The listing builds one solid part. Answer for the finished solid, in the listing's coordinates (mm). A direction names the side the tool comes from. Give positions to 0.01 mm unless a question says otherwise; leave off trailing zeros. Loops run counter-clockwise (first coordinate to the right, second up) from the corner with the lowest first, then second, coordinate; pieces in that order, holes last. Notation, with made-up numbers: (27.25, -1.75) - (86.25, -1.75) arc R17 ccw to (86.25, 16.25) - close; hole circle Ø5 at (35, 81). An arc over 180 degrees is marked (long way). One line per item, written item: value. Start each with the question number.
from build123d import *

# Parameters (mm, degrees)
CYLINDER026_R     = 1.75
CYLINDER026_DEPTH = 20
CYLINDER025_R     = 1.75
CYLINDER025_DEPTH = 20
CYLINDER014_R     = 1.2
CYLINDER014_DEPTH = 10
CYLINDER013_R     = 1.2
CYLINDER013_DEPTH = 10
SKETCH_R          = 4
PAD_DEPTH         = 3
BOX008_W          = 23.5
BOX008_H          = 12.5
BOX008_DEPTH      = 10
BOX007_W          = 32.5
BOX007_H          = 12.5
BOX007_DEPTH      = 2
BOX006_W          = 40.5
BOX006_H          = 20.5
BOX006_DEPTH      = 9.5


with BuildPart() as cylinder061:
    # Cylinder026 → Cylinder026 (new body)
    with BuildSketch(Plane(origin=(40, -18, 77), x_dir=(1, 0, 0), z_dir=(0, 0, 1))):
        Circle(CYLINDER026_R)
    extrude(amount=CYLINDER026_DEPTH)


with BuildPart() as cylinder060:
    # Cylinder025 → Cylinder025 (new body)
    with BuildSketch(Plane(origin=(28, -18, 77), x_dir=(1, 0, 0), z_dir=(0, 0, 1))):
        Circle(CYLINDER025_R)
    extrude(amount=CYLINDER025_DEPTH)


with BuildPart() as cylinder049:
    # Cylinder014 → Cylinder014 (new body)
    with BuildSketch(Plane(origin=(55, 19, -5), x_dir=(1, 0, 0), z_dir=(0, 0, 1))):
        Circle(CYLINDER014_R)
    extrude(amount=CYLINDER014_DEPTH)


with BuildPart() as cylinder048:
    # Cylinder013 → Cylinder013 (new body)
    with BuildSketch(Plane(origin=(55, -9.5, -5), x_dir=(1, 0, 0), z_dir=(0, 0, 1))):
        Circle(CYLINDER013_R)
    extrude(amount=CYLINDER013_DEPTH)


with BuildPart() as tapa:
    # Sketch → Pad (new body)
    with BuildSketch(Plane.XY.offset(-3)):
        with BuildLine():
            ThreePointArc((13.733879, 10.914307), (6.136168, -2.245404), (17.776624, -12.012848))
            Line((17.776624, -12.012848), (97.776624, -12.012848))
            ThreePointArc((97.776624, -12.012848), (119.712869, 11.926287), (93.95296, 31.692625))
            Line((13.733879, 10.914307), (93.95296, 31.692625))
        make_face()
        with Locations((17.77659, -0.192848)):
            Circle(SKETCH_R, mode=Mode.SUBTRACT)
        with Locations((97.776659, 10.007152)):
            Circle(SKETCH_R, mode=Mode.SUBTRACT)
    extrude(amount=PAD_DEPTH)


with BuildPart() as cube008:
    # Box008 → Box008 (new body)
    with BuildSketch(Plane(origin=(8.5, 4, 0), x_dir=(1, 0, 0), z_dir=(0, 0, 1))):
        with Locations((11.75, 6.25)):
            Rectangle(BOX008_W, BOX008_H)
    extrude(amount=BOX008_DEPTH)


with BuildPart() as cube007:
    # Box007 → Box007 (new body)
    with BuildSketch(Plane(origin=(4, 4, 0), x_dir=(1, 0, 0), z_dir=(0, 0, 1))):
        with Locations((16.25, 6.25)):
            Rectangle(BOX007_W, BOX007_H)
    extrude(amount=BOX007_DEPTH)


with BuildPart() as tapa_izquierda_interior:
    # Box006 → Box006 (new body)
    with BuildSketch(Plane.XY):
        with Locations((20.25, 10.25)):
            Rectangle(BOX006_W, BOX006_H)
    extrude(amount=BOX006_DEPTH)

    # Cut008: cut Cube007
    add(cube007.part, mode=Mode.SUBTRACT)

    # Cut009: cut Cube008
    add(cube008.part, mode=Mode.SUBTRACT)


with BuildPart() as tapa_izquierda_interior_1:
    # Cut009 placement: moved
    add(tapa_izquierda_interior.part.moved(Location((72.5, 0, -12.5))))

    # Fusion006: union Tapa
    add(tapa.part)


with BuildPart() as tapa_izquierda_interior_2:
    # Fusion006 placement: moved
    add(tapa_izquierda_interior_1.part.moved(Location((0, 0, -0.5))))

    # Cut013: cut Cylinder048
    add(cylinder048.part, mode=Mode.SUBTRACT)

    # Cut014: cut Cylinder049
    add(cylinder049.part, mode=Mode.SUBTRACT)


with BuildPart() as tapa_izquierda_interior_3:
    # Cut014 placement: moved
    add(tapa_izquierda_interior_2.part.moved(Location((-21, -19, 89))))

    # Cut049: cut Cylinder060
    add(cylinder060.part, mode=Mode.SUBTRACT)

    # Cut050: cut Cylinder061
    add(cylinder061.part, mode=Mode.SUBTRACT)


solid = tapa_izquierda_interior_3.part
1. A cutting plane is placed at B-B (x = 34). Determine the outline of the cut face in (y, z).
2. Flat-ended cylindrical pins translate along their axes: pin 1 (5 mm diameter, centred on x = 71, z = 80.5, fed in from +Y); pin 2 (6 mm diameter, centred on y = -24.5, z = 86, fed in from -X); pin 3 (3 mm diameter, centred on y = -19, z = 83, fed in from -X). Find the tip coordinate at first contact, or state that the pin passes through.
3. Determine the mould class of faces 1 (the flat face through (32.282, 2.158, 86.979)), 2 (the cylindrical face through (40.9, -16.5, 87)), 3 (the cylindrical face through (72.78, -8.82, 86.98)), 4 (the flat face through (36, -31.013, 87)) for opening direction X: released by +X, released by -X, zero draft, split by the parting line, or undercut.
4. A cutting plane is placed at A-A (z = 80). Determine the outline of the cut face in (x, y), plus the area to 4 significant figures.
5. Find the intervals of material crossed by L1, parallel to X at y = -18, z = 86.35; L2, parallel to Y at x = 34, z = 86.6; L3, parallel to Y at x = 78, z = 77.25, in increasing order. Write a range as [from, to].
6. For faces 5 (the flat face through (51.5, -9, 81)), 6 (the cylindrical face through (-14.9, -21.02, 86.98)), 7 (the flat face through (71, 1.5, 81)), 8 (the flat face through (92, -9, 81)), 9 (the flat face through (72, -15, 81)), determine the directions among +Z, -Z, +X, -X, +Y, -Y from which every point of the face is accessible in a straight line to the end or side of a thin tool.
7. A cutting plane is placed at D-D (x = -1). Determine the outline of the cut face in (y, z), plus the area to 3 significant figures.
8. A cutting plane is placed at C-C (y = -12). Determine the outline of the cut face in (x, z), plus the area to 3 significant figures.
Results below:
1. outline: (-31.01, 85.5) - (-29.7, 85.5) - (-29.7, 88.5) - (-31.01, 88.5) - close; (-27.3, 85.5) - (-1.2, 85.5) - (-1.2, 88.5) - (-27.3, 88.5) - close; (1.2, 85.5) - (2.6, 85.5) - (2.6, 88.5) - (1.2, 88.5) - close
2. pin 1: stops at y = 1.5
2. pin 2: stops at x = -14.82
2. pin 3: stops at x = 51.5
3. face 1: released by -X
3. face 2: undercut
3. face 3: undercut
3. face 4: zero draft
4. outline: (51.5, -19) - (92, -19) - (92, 1.5) - (51.5, 1.5) - close; hole (60, -15) - (83.5, -15) - (83.5, -2.5) - (60, -2.5) - close
4. area: 536.5 mm^2
5. L1: x = [-14.98, -7.04], [0.59, 26.25], [29.75, 38.25], [41.75, 96.87]
5. L2: y = [-31.01, -29.7], [-27.3, -1.2], [1.2, 2.6]
5. L3: y = [-19, -15], [-2.5, 1.5]
6. face 5: -Z, -X, +Y, -Y
6. face 6: +Z, -Z, -X
6. face 7: -Z, +X, -X, +Y
6. face 8: -Z, +X, +Y, -Y
6. face 9: -Z
7. outline: (-31.01, 85.5) - (-22.52, 85.5) - (-22.52, 88.5) - (-31.01, 88.5) - close; (-15.87, 85.5) - (-6.46, 85.5) - (-6.46, 88.5) - (-15.87, 88.5) - close
7. area: 53.7 mm^2
8. outline: (-12.6, 85.5) - (51.5, 85.5) - (51.5, 76) - (55.5, 76) - (55.5, 78) - (60, 78) - (60, 85.5) - (74.14, 85.5) - (74.14, 88.5) - (-12.6, 88.5) - close; (79.41, 85.5) - (83.5, 85.5) - (83.5, 78) - (88, 78) - (88, 76) - (92, 76) - (92, 85.5) - (98.59, 85.5) - (98.59, 88.5) - (79.41, 88.5) - close
8. area: 461 mm^2
